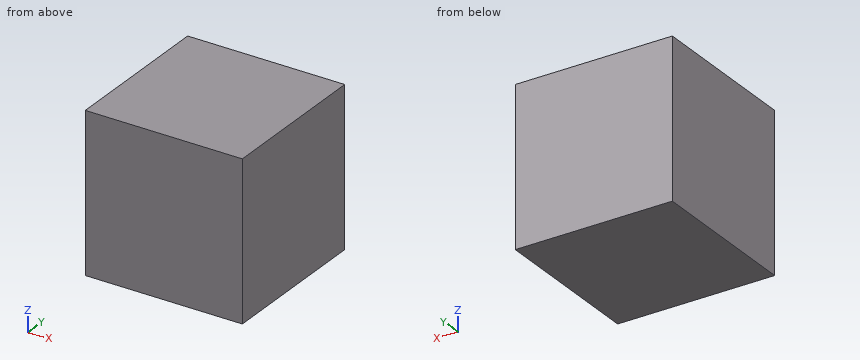
```python
from build123d import *

# Parameters (mm, degrees)
F0_W     = 20
F0_H     = 20
F1_DEPTH = 10
F2_T     = -1


with BuildPart() as f1:
    # F0 (on Front) → F1 (new body, symmetric)
    with BuildSketch(Plane.XZ):
        Rectangle(F0_W, F0_H)
    extrude(amount=F1_DEPTH, both=True)

    # F2 (hollow: no face is removed)
    offset(amount=F2_T, mode=Mode.SUBTRACT)


solid = f1.part
```
Read the model definition and answer for the solid it produces. Units are mm, in the model's axes. Coordinates: 2 decimals unless noted, no trailing zeros. Loops run counter-clockwise (first coordinate to the right, second up) from the corner with the lowest first, then second, coordinate; pieces in that order, holes last. Notation, with made-up numbers: (-9, 64.25) -> (-5, 64.25) arc R27 ccw to (-5, 101.25) -> close; hole circle Ø9 at (16.5, 70). An arc over 180 degrees is marked (long way). Return JSON: item names as keys, results as strings.
Item 1: Find section A-A (z = -2.5). Determine the outline of the cut face in (x, y).
Answers:
{"outline": "(-10, -10) -> (10, -10) -> (10, 10) -> (-10, 10) -> close; hole (-9, -9) -> (9, -9) -> (9, 9) -> (-9, 9) -> close"}
Item 2: Find the intervals of material crossed by probe 1 along Z at (x, y) = (1.75, 6.5), in increasing order.
Answers:
{"probe 1": "z = -10 to -9, 9 to 10"}
